Can you work these out from the drawing? Everything is in mm from the part's minimum corner. A direction names the side the tool comes from. Round coordinates to 2 decimals unless told otherwise and drop trailing zeros. Loops run counter-clockwise (first coordinate to the right, second up) from the corner with the lowest first, then second, coordinate; pieces in that order, holes last. Notation, with made-up numbers: M 62,61 L 68,61 A34 ccw 68,99 Z; hole C 81,-10 d4. An arc over 180 degrees is marked long. Answer in a Markdown table with one row per item.
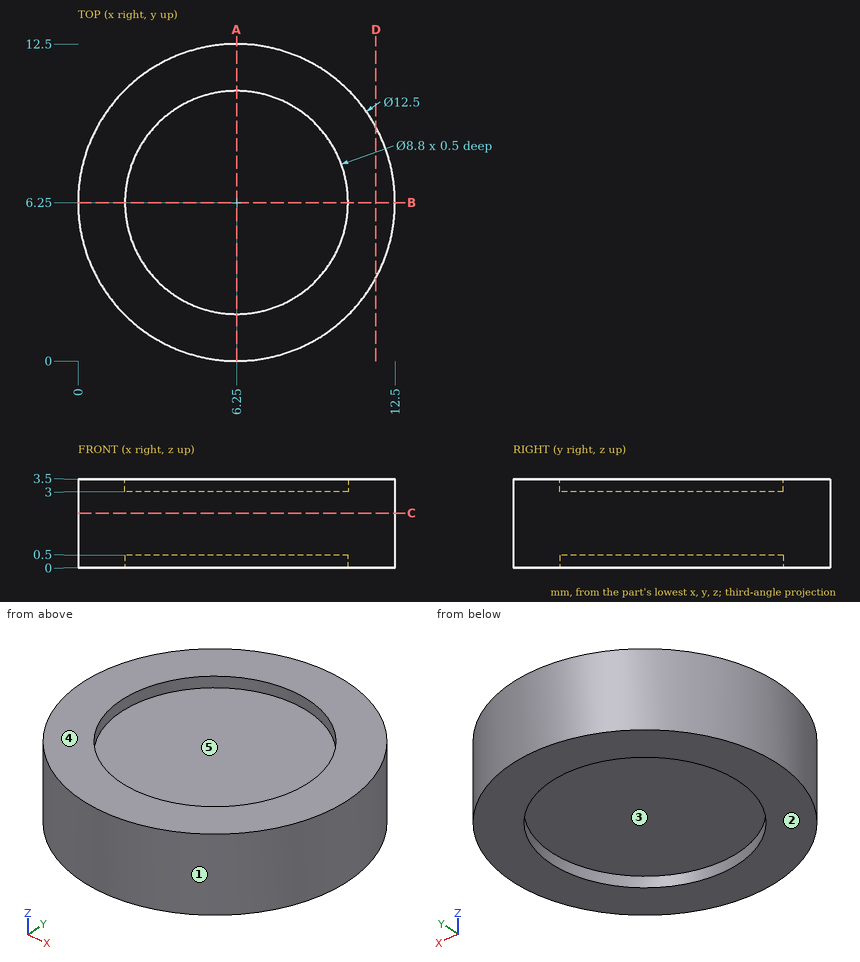
1) I want a section at A-A, the plane x = 6.25. Please give me the cut outline in (y, z).
Computed:
| item | result |
|---|---|
| outline | M 0,0 L 1.85,0 L 1.85,0.5 L 10.65,0.5 L 10.65,0 L 12.5,0 L 12.5,3.5 L 10.65,3.5 L 10.65,3 L 1.85,3 L 1.85,3.5 L 0,3.5 Z |
2) Which directions (+Z, -Z, +X, -X, +Y, -Y) give clear straight access to the entire face, cutting with the end or side of a thin tool? Please do the marked faces 4 and 5.
Computed:
| item | result |
|---|---|
| face 4 | +Z, +X, -X, +Y, -Y |
| face 5 | +Z |
3) I need wall thicknesses on line 1 (Y direction, x = 6.25, z = 0.3); line 2 (Z direction, x = 5.75, y = 7.5); line 3 (X direction, y = 4.75, z = 3.2). Which ranges of each line are inside material? Lowest first, please.
Computed:
| item | result |
|---|---|
| line 1 | y = 0 to 1.85, 10.65 to 12.5 |
| line 2 | z = 0.5 to 3 |
| line 3 | x = 0.18 to 2.11, 10.39 to 12.32 |
4) I want a section at D-D, the plane x = 11.75. Please give me the cut outline in (y, z).
Computed:
| item | result |
|---|---|
| outline | M 3.28,0 L 9.22,0 L 9.22,3.5 L 3.28,3.5 Z |
5) I want a section at C-C, the plane z = 2.15. Please give me the cut outline in (x, y).
Computed:
| item | result |
|---|---|
| outline | C 6.25,6.25 d12.5 |
6) Will these pins go through, and if not, where does the flat tip stop? P1, Ø2, axis at y = 5, z = 1, coming from the +X side (3 decimals); P2, Ø3, axis at x = 3, y = 8, coming from the -Z side; P3, Ø2.5, axis at x = 7.5, y = 7, coming from the -Z side; P4, Ø2, axis at y = 9.5, z = 0.5, coming from the -X side.
Computed:
| item | result |
|---|---|
| P1 | stops at x = 12.495 |
| P2 | stops at z = 0 |
| P3 | stops at z = 0.5 |
| P4 | stops at x = 0.42 |
7) If we mould it in two halves opening along Y, with no side actions, what happens to the marked faces 1, 2 and 3? For each: released by +Y, released by -Y, zero draft, split by the parting line, or undercut.
Computed:
| item | result |
|---|---|
| face 1 | split by the parting line |
| face 2 | zero draft |
| face 3 | undercut |
